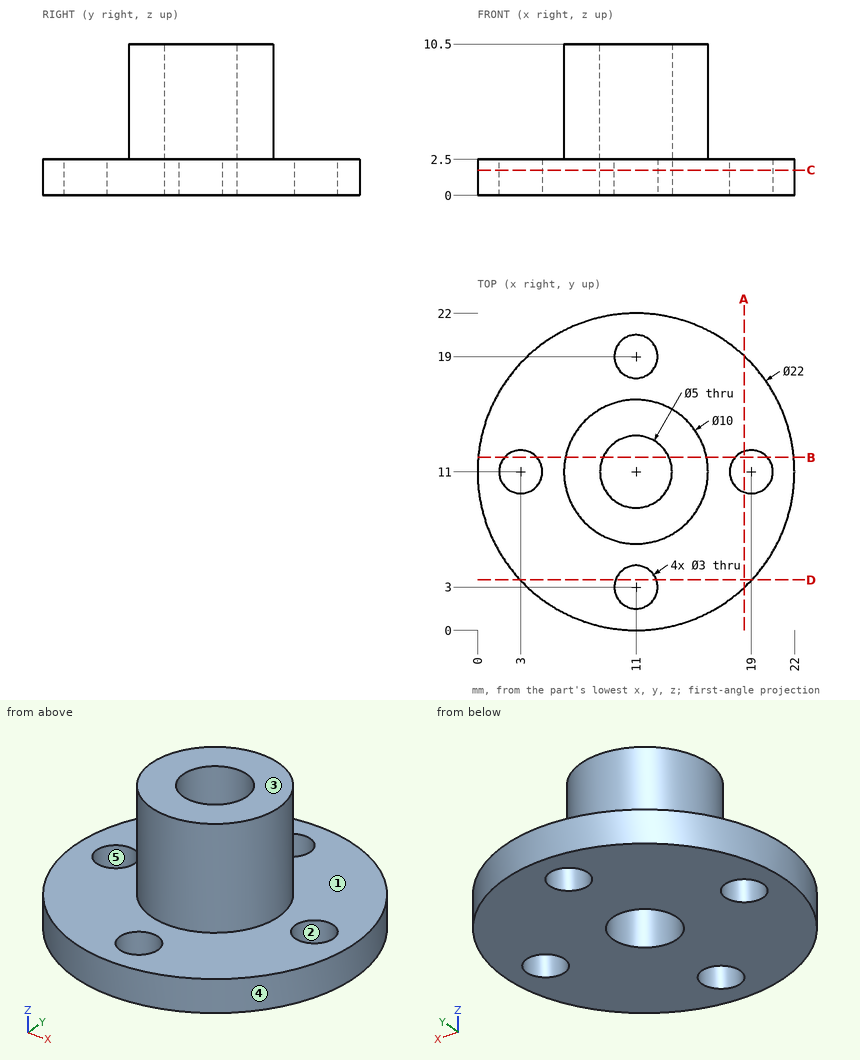
Design review of the part shown in the three views and the two pictorial views. Dimensions are in mm from the part's minimum x, y and z. A direction names the side the tool comes from. Round coordinates to 2 decimals unless told otherwise and drop trailing zeros. Order: outer loops, then holes, each group sorted by start corner. A loop starts at its lowest first (then second) coordinate and runs counter-clockwise, first axis right, second up. Notation, with made-up numbers: (31.25, 62) -> (85.25, 62) arc R18 ccw to (85.25, 86) -> close; hole circle Ø3 at (33.5, 37). An arc over 180 degrees is marked (long way). Write item = value, one per line. Start each with the question number.
1) Insertion check: pin 1 (2 mm diameter, centred on x = 16, z = 8, fed in from +Y); pin 2 (5 mm diameter, centred on x = 11, y = 19, fed in from +Z). Each pin has a flat end and moves straight along its axis. Give the tip position at first contact, or say it passes through.
2) Take a section at C-C on z = 1.75. State the section outline as (x, y) points, plus the area to 3 significant figures.
3) To check wall thickness, follow line 1 (Y direction, x = 11, z = 0.55); line 2 (Z direction, x = 8, y = 5.5); line 3 (Y direction, x = 11, z = 4.25). State the ranges of each line that lie inside material, in increasing order. Write a range as from..to.
4) Take a section at A-A on x = 18.5. State the section outline as (y, z) points.
5) Tool access review of the marked faces 1 and 2: name each direction out of +Z, -Z, +X, -X, +Y, -Y from which nothing blocks a thin tool from reaching the whole face with its end or side.
6) Take a section at B-B on y = 12. State the section outline as (x, z) points.
7) The part is to be moulded in two halves that separate along Y. For the marked faces 3, 4 and 5, say which applies: +Y half, -Y half, draft (parallel to the pull), parting line (faces both ways), or undercut.
Verdict:
q1.pin_1 = 14
q1.pin_2 = 2.5
q2.outline = circle Ø22 at (11, 11); hole circle Ø3 at (3, 11); hole circle Ø5 at (11, 11); hole circle Ø3 at (11, 3); hole circle Ø3 at (11, 19); hole circle Ø3 at (19, 11)
q2.area = 332 mm2
q3.line_1 = 0..1.5, 4.5..8.5, 13.5..17.5, 20.5..22
q3.line_2 = 0..2.5
q3.line_3 = 6..8.5, 13.5..16
q4.outline = (2.95, 0) -> (9.59, 0) -> (9.59, 2.5) -> (2.95, 2.5) -> close; (12.41, 0) -> (19.05, 0) -> (19.05, 2.5) -> (12.41, 2.5) -> close
q5.face_1 = +Z
q5.face_2 = +Z, -Z
q6.outline = (0.05, 0) -> (1.88, 0) -> (1.88, 2.5) -> (0.05, 2.5) -> close; (4.12, 0) -> (8.71, 0) -> (8.71, 10.5) -> (6.1, 10.5) -> (6.1, 2.5) -> (4.12, 2.5) -> close; (13.29, 0) -> (17.88, 0) -> (17.88, 2.5) -> (15.9, 2.5) -> (15.9, 10.5) -> (13.29, 10.5) -> close; (20.12, 0) -> (21.95, 0) -> (21.95, 2.5) -> (20.12, 2.5) -> close
q7.face_3 = draft
q7.face_4 = parting line
q7.face_5 = undercut
